```python
from build123d import *

# Parameters (mm, degrees)
ESQUISSE1_W             = 16.999166609
ESQUISSE1_H             = 11.2
ESQUISSE1_R             = 1.75
BOSS_EXTRU_1_DEPTH      = 5
ESQUISSE2_W             = 2
ESQUISSE2_H             = 7.2
BOSS_EXTRU_2_DEPTH      = 20
ESQUISSE3_W             = 4
ESQUISSE3_H             = 7.2
ENL_V_MAT_EXTRU_1_DEPTH = 20
ESQUISSE4_R             = 1.25
ESQUISSE4_W             = 4.999166609
ESQUISSE4_H             = 20
ENL_V_MAT_EXTRU_2_DEPTH = 20
ESQUISSE5_R             = 2.95
ENL_V_MAT_EXTRU_3_DEPTH = 2.5
CONG_1_START            = -11.2
CONG_1_DEPTH            = 12.2
CONG_1_2_DEPTH          = 2
CONG_1_START_2          = -2
CONG_1_3_DEPTH          = 2


with BuildPart() as part:
    # Esquisse1 → Boss.-Extru.1 (new body)
    with BuildSketch(Plane.XY):
        with Locations((8.499583304, -5.6)):
            Rectangle(ESQUISSE1_W, ESQUISSE1_H)
        with Locations((5.5, -5.6)):
            Circle(ESQUISSE1_R, mode=Mode.SUBTRACT)
        with Locations((11.499166609, -5.5)):
            Circle(ESQUISSE1_R, mode=Mode.SUBTRACT)
    extrude(amount=BOSS_EXTRU_1_DEPTH)

    # Esquisse2 → Boss.-Extru.2 (add)
    with BuildSketch(Plane.XY.offset(5)):
        Polygon((14.999166609, -9.2), (0, -9.2), (0, -11.2), (16.999166609, -11.2), (16.999166609, -9.2), align=None)
        with Locations((15.999166609, -5.6)):
            Rectangle(ESQUISSE2_W, ESQUISSE2_H)
        Polygon((16.999166609, 0), (0, 0), (0, -2), (14.999166609, -2), (16.999166609, -2), align=None)
    extrude(amount=BOSS_EXTRU_2_DEPTH)

    # Esquisse3 → Enlèv. mat.-Extru.1 (cut)
    with BuildSketch(Plane.ZY.offset(-14.999166609)):
        with Locations((7, -5.6)):
            Rectangle(ESQUISSE3_W, ESQUISSE3_H)
        with Locations((23, -5.6)):
            Rectangle(ESQUISSE3_W, ESQUISSE3_H)
        with Locations((16, -5.6)):
            Rectangle(ESQUISSE3_W, ESQUISSE3_H)
    extrude(amount=-ENL_V_MAT_EXTRU_1_DEPTH, mode=Mode.SUBTRACT)

    # Esquisse4 → Enlèv. mat.-Extru.2 (cut)
    with BuildSketch(Plane(origin=(0, -11.2, 0), x_dir=(-1, 0, 0), z_dir=(0, -1, 0))):
        with Locations(Location((-11.499166609, -20, 0), (0, 0, 90))):
            Circle(ESQUISSE4_R)
        with Locations(Location((-11.499166609, -10.5, 0), (0, 0, 90))):
            Circle(ESQUISSE4_R)
        with Locations((-2.499583305, -15)):
            Rectangle(ESQUISSE4_W, ESQUISSE4_H)
    extrude(amount=-ENL_V_MAT_EXTRU_2_DEPTH, mode=Mode.SUBTRACT)

    # Esquisse5 → Enlèv. mat.-Extru.3 (cut)
    with BuildSketch(Plane.XY.offset(5)):
        with Locations((5.5, -5.6)):
            Circle(ESQUISSE5_R)
        with Locations((11.499166609, -5.5)):
            Circle(ESQUISSE5_R)
    extrude(amount=-ENL_V_MAT_EXTRU_3_DEPTH, mode=Mode.SUBTRACT)

    # Congé1: read off the stored shape, not the designer's step
    # Congé1 outline → Congé1 (cut)
    with BuildSketch(Plane(origin=(0, 0, 0), x_dir=(1, 0, 0), z_dir=(0, 1, 0)).offset(CONG_1_START)):
        with BuildLine():
            ThreePointArc((7.999166609, -25), (5.877846265, -24.121320344), (4.999166609, -22))
            Line((4.999166609, -22), (4.999166609, -25))
            Line((4.999166609, -25), (7.999166609, -25))
        make_face()
    extrude(amount=CONG_1_DEPTH, mode=Mode.SUBTRACT)

    # Cong_1 2 outline → Cong_1 2 (add)
    with BuildSketch(Plane(origin=(0, 0, 0), x_dir=(1, 0, 0), z_dir=(0, 1, 0)).offset(CONG_1_START)):
        with BuildLine():
            ThreePointArc((1.999166609, -5), (4.120486952, -5.878679656), (4.999166609, -8))
            Line((4.999166609, -8), (4.999166609, -5))
            Line((4.999166609, -5), (1.999166609, -5))
        make_face()
    extrude(amount=CONG_1_2_DEPTH)

    # Cong_1 3 outline → Cong_1 3 (add)
    with BuildSketch(Plane(origin=(0, 0, 0), x_dir=(1, 0, 0), z_dir=(0, 1, 0)).offset(CONG_1_START_2)):
        with BuildLine():
            ThreePointArc((1.999166609, -5), (4.120486952, -5.878679656), (4.999166609, -8))
            Line((4.999166609, -8), (4.999166609, -5))
            Line((4.999166609, -5), (1.999166609, -5))
        make_face()
    extrude(amount=CONG_1_3_DEPTH)


solid = part.part
```
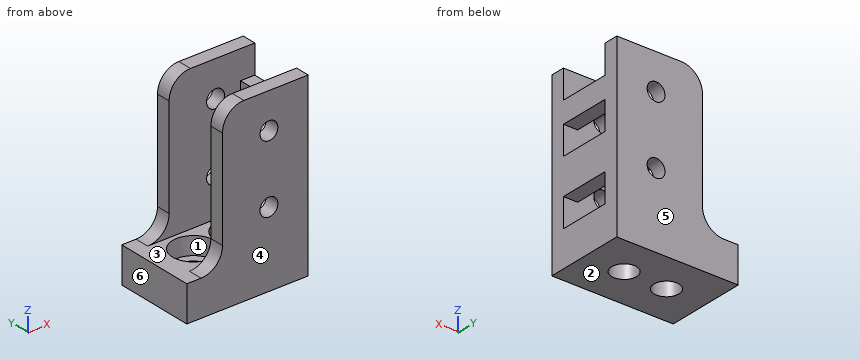
Geometry: final body of the model. Coordinates: model frame, mm. Face numbers are marked on the shaded views. A direction names the side the tool comes from. Coordinates: 2 decimals unless noted, no trailing zeros. Order: outer loops, then holes, each group sorted by start corner. A loop starts at its lowest first (then second) coordinate and runs counter-clockwise, first axis right, second up. Notation, with made-up numbers: (24.5, 72.5) -> (81.5, 72.5) arc R19 ccw to (81.5, 82.5) -> close; hole circle Ø3 at (56.5, 73). An arc over 180 degrees is marked (long way). Answer in a Markdown table with one row per item.
Item 1: Access query for the marked faces 1 and 2. Directions: +Z, -Z, +X, -X, +Y, -Y. A direction counts if a zero-diameter tool reaches every point of the face in a straight line with its end or side. Return the directions, or none.
Return value:
| item | result |
|---|---|
| face 1 | +Z |
| face 2 | -Z, +X, -X, +Y, -Y |
Item 2: Ray query, L1, parallel to Z at x = 16, y = -7; L2, parallel to X at y = -5.6, z = 1.2. Return the intervals inside material, ascending.
Return value:
| item | result |
|---|---|
| L1 | z = 0 to 5, 9 to 14, 18 to 21 |
| L2 | x = 0 to 3.75, 7.25 to 9.75, 13.25 to 17 |
Item 3: Section C-C on z = 4. Output: boundary loops of the cut face in (x, y).
Return value:
| item | result |
|---|---|
| outline | (0, -11.2) -> (17, -11.2) -> (17, 0) -> (0, 0) -> close; hole circle Ø5.9 at (5.5, -5.6); hole circle Ø5.9 at (11.5, -5.5) |
Item 4: Draft query along Y for the marked faces 3, 4, 5 and 6. Return one class per face: released by +Y, released by -Y, zero draft, split by the parting line, or undercut.
Return value:
| item | result |
|---|---|
| face 3 | undercut |
| face 4 | released by -Y |
| face 5 | released by +Y |
| face 6 | zero draft |
Item 5: Contact query for flat-ended pins moving along their axis: P1, Ø1.5, axis at y = -6.5, z = 10.5, coming from the -X side; P2, Ø6.5, axis at x = 4.5, y = -4, coming from the +Z side; P3, Ø1, axis at y = -3, z = 16, coming from the -X side; P4, Ø1, axis at x = 16, y = -7, coming from the +Z side. Output: stop coordinate, or through.
Return value:
| item | result |
|---|---|
| P1 | stops at x = 15 |
| P2 | stops at z = 24.85 |
| P3 | passes through |
| P4 | stops at z = 21 |
Item 6: Section D-D on y = -1. Output: boundary loops of the cut face in (x, z), plus the area to 3 significant figures.
Return value:
| item | result |
|---|---|
| outline | (0, 0) -> (17, 0) -> (17, 25) -> (8, 25) arc R3 ccw to (5, 22) -> (5, 8) arc R3 cw to (2, 5) -> (0, 5) -> close; hole circle Ø2.5 at (11.5, 10.5); hole circle Ø2.5 at (11.5, 20) |
| area | 315 mm² |
Item 7: Section A-A on z = 10.5. Output: boundary loops of the cut face in (x, y), plus the area to 3 significant figures.
Return value:
| item | result |
|---|---|
| outline | (5, -11.2) -> (10.25, -11.2) -> (10.25, -9.2) -> (5, -9.2) -> close; (5, -2) -> (10.25, -2) -> (10.25, 0) -> (5, 0) -> close; (12.75, -11.2) -> (17, -11.2) -> (17, 0) -> (12.75, 0) -> (12.75, -2) -> (15, -2) -> (15, -9.2) -> (12.75, -9.2) -> close |
| area | 52.4 mm² |
Item 8: Section B-B on y = -6. Output: boundary loops of the cut face in (x, z), plus the area to 3 significant figures.
Return value:
| item | result |
|---|---|
| outline | (0, 0) -> (3.8, 0) -> (3.8, 2.5) -> (2.58, 2.5) -> (2.58, 5) -> (0, 5) -> close; (7.2, 0) -> (9.82, 0) -> (9.82, 2.5) -> (8.59, 2.5) -> (8.59, 5) -> (8.42, 5) -> (8.42, 2.5) -> (7.2, 2.5) -> close; (13.18, 0) -> (17, 0) -> (17, 5) -> (14.41, 5) -> (14.41, 2.5) -> (13.18, 2.5) -> close; (15, 9) -> (17, 9) -> (17, 14) -> (15, 14) -> close; (15, 18) -> (17, 18) -> (17, 21) -> (15, 21) -> close |
| area | 54.9 mm² |
